Here's the drawing with two shaded views (mm, measured from the low corner). I have some questions. Round coordinates to 2 decimals unless told otherwise and drop trailing zeros. Loops run counter-clockwise (first coordinate to the right, second up) from the corner with the lowest first, then second, coordinate; pieces in that order, holes last. Notation, with made-up numbers: (42, 59.5) - (79, 59.5) arc R20 ccw to (79, 73.5) - close; hole circle Ø1 at (-31, -25.75). An arc over 180 degrees is marked (long way). Use one line per item in the form item = value.
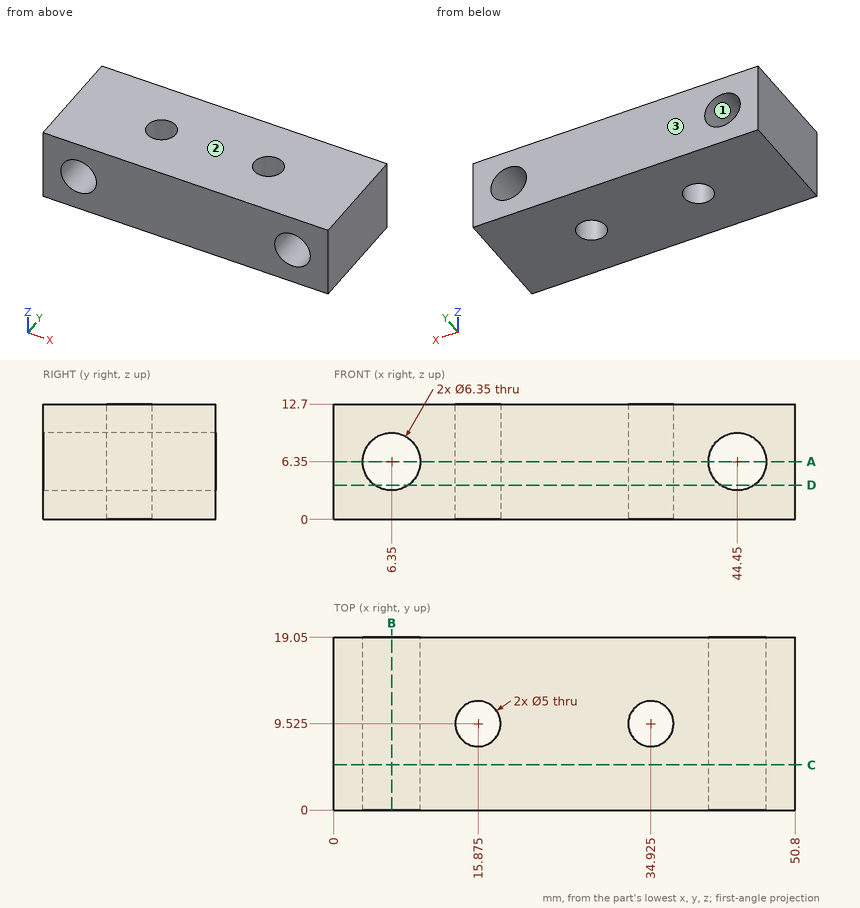
1. If we section it at B-B, the plane x = 6.35: Write out the boundary of the cut face in (y, z) (3 decimals).
Solution:
outline = (0, 0) - (19.05, 0) - (19.05, 3.175) - (0, 3.175) - close; (0, 9.525) - (19.05, 9.525) - (19.05, 12.7) - (0, 12.7) - close
2. If we section it at C-C, the plane y = 5: Write out the boundary of the cut face in (x, z) (3 decimals).
Solution:
outline = (0, 0) - (50.8, 0) - (50.8, 12.7) - (0, 12.7) - close; hole circle Ø6.35 at (6.35, 6.35); hole circle Ø6.35 at (44.45, 6.35)
3. We'd pull the mould along Z, two halves only. Please class the marked faces 1, 2 and 3: +Z half, -Z half, draft (parallel to the pull), parting line (faces both ways), or undercut.
Solution:
face_1 = undercut
face_2 = +Z half
face_3 = draft
4. Please list where these lines run through material, in increasing order: line 1 along X through (y, z) = (14.75, 6.35) (3 decimals); line 2 along Y through (x, z) = (16, 12); line 3 along X through (y, z) = (9.25, 4).
Solution:
line_1 = 0 to 3.175, 9.525 to 41.275, 47.625 to 50.8
line_2 = 0 to 7.03, 12.02 to 19.05
line_3 = 0 to 4.22, 8.48 to 13.39, 18.36 to 32.44, 37.41 to 42.32, 46.58 to 50.8
5. If we section it at D-D, the plane z = 3.75: Write out the boundary of the cut face in (x, y) (3 decimals).
Solution:
outline = (0, 0) - (4.528, 0) - (4.528, 19.05) - (0, 19.05) - close; (8.172, 0) - (42.628, 0) - (42.628, 19.05) - (8.172, 19.05) - close; (46.272, 0) - (50.8, 0) - (50.8, 19.05) - (46.272, 19.05) - close; hole circle Ø5 at (15.875, 9.525); hole circle Ø5 at (34.925, 9.525)
6. If we section it at A-A, the plane z = 6.35: Write out the boundary of the cut face in (x, y) (3 decimals), plus the area to 3 significant figures.
Solution:
outline = (0, 0) - (3.175, 0) - (3.175, 19.05) - (0, 19.05) - close; (9.525, 0) - (41.275, 0) - (41.275, 19.05) - (9.525, 19.05) - close; (47.625, 0) - (50.8, 0) - (50.8, 19.05) - (47.625, 19.05) - close; hole circle Ø5 at (15.875, 9.525); hole circle Ø5 at (34.925, 9.525)
area = 687 mm^2
7. For P1, Ø4, axis at x = 34.925, y = 9.525, coming from the +Z side, with a flat end and sliding along its axis, tell me the tip position at first contact or that it passes through.
Solution:
P1 = through
